```python
from build123d import *

# Parameters (mm, degrees)
EXTRUDE_11_REACH             = 60.31
EXTRUDE_11_DIRECTION_2_REACH = 60.31
CUT_EXTRUDE_1_DEPTH          = 7.5
CUT_EXTRUDE_1_DEPTH_BACK     = 7.5
CUT_EXTRUDE_2_DEPTH          = 5
CUT_EXTRUDE_START            = 28.688718626
CUT_EXTRUDE_3_DEPTH          = 1.311276176


# Read off the part's stored shape, not the designer's step: 切除-拉伸3
with BuildPart() as part:
    # 草图1 → 旋转1 (revolve)
    with BuildSketch(Plane.XY, mode=Mode.PRIVATE) as revolve_1_sk:
        Polygon((26.5, 38.4), (26.5, 36), (29, 36), (29, 0), (30, 0), (30, 40), (29, 40), (29, 38.4), align=None)
    revolve_1 = revolve(revolve_1_sk.sketch.rotate(Axis((0, 66, 0), (0, -1, 0)), 90), axis=Axis((0, 66, 0), (0, -1, 0)))

    # 镜向1: 旋转1 across plane
    add(revolve_1.mirror(Plane.ZX))

    # 凸台-拉伸11: up to this face of the body (flat: up to its plane)
    extrude_11_end = Plane(part.part.faces().sort_by_distance((0, 36, -27.320243866))[0])
    # 草图11 → 凸台-拉伸11 (add, up to the picked face)
    with BuildSketch(Plane(origin=(0, 0, 0), x_dir=(1, 0, 0), z_dir=(0, 1, 0)), mode=Mode.PRIVATE) as extrude_11_sk1:
        with BuildLine():
            Line((-13.076696831, -27), (13.076696831, -27))
            ThreePointArc((13.076696831, -27), (0, -30), (-13.076696831, -27))
        make_face()
    extrude_11_tool1 = split(extrude(extrude_11_sk1.sketch, amount=EXTRUDE_11_REACH, mode=Mode.PRIVATE), bisect_by=extrude_11_end, keep=Keep.BOTH, mode=Mode.PRIVATE)
    add(extrude_11_tool1.solids().sort_by(Axis((0, 0, 28.205296), (0, 1, 0)))[0])

    # 凸台-拉伸11 direction 2: up to this face of the body (flat: up to its plane)
    extrude_11_direction_2_end = Plane(part.part.faces().sort_by_distance((0, -36, -27.320243866))[0])
    # 草图11 → 凸台-拉伸11 direction 2 (add, up to the picked face)
    with BuildSketch(Plane(origin=(0, 0, 0), x_dir=(1, 0, 0), z_dir=(0, 1, 0)), mode=Mode.PRIVATE) as extrude_11_direction_2_sk1:
        with BuildLine():
            Line((-13.076696831, -27), (13.076696831, -27))
            ThreePointArc((13.076696831, -27), (0, -30), (-13.076696831, -27))
        make_face()
    extrude_11_direction_2_tool1 = split(extrude(extrude_11_direction_2_sk1.sketch, amount=-EXTRUDE_11_DIRECTION_2_REACH, mode=Mode.PRIVATE), bisect_by=extrude_11_direction_2_end, keep=Keep.BOTH, mode=Mode.PRIVATE)
    add(extrude_11_direction_2_tool1.solids().sort_by(Axis((0, 0, 28.205296), (0, -1, 0)))[0])

    # 草图12 → 切除-拉伸1 (cut, two sides: drawn at the far end of the back side and taken through both)
    with BuildSketch(Plane(origin=(0, 0, 0), x_dir=(1, 0, 0), z_dir=(0, 1, 0)).offset(-CUT_EXTRUDE_1_DEPTH_BACK)):
        with BuildLine():
            Line((0, 0), (22.520337054, 22.934948885))
            ThreePointArc((22.520337054, 22.934948885), (31.296937417, -7.32660697), (10, -30.547953473))
            Line((10, -30.547953473), (0, 0))
        make_face()
    extrude(amount=CUT_EXTRUDE_1_DEPTH + CUT_EXTRUDE_1_DEPTH_BACK, mode=Mode.SUBTRACT)

    # Sketch 3D_2 → 切除-拉伸2 (cut)
    with BuildSketch(Plane(origin=(35, 15, -4.993961669), x_dir=(-0.989973390659655, 0, 0.1412539761770484), z_dir=(0, 1, 0))):
        with BuildLine():
            Line((0, 0), (35.354485616, 0))
            Line((35.354485616, 0), (0.330334968, 4.976372773))
            ThreePointArc((0.330334968, 4.976372773), (0.075684949, 2.494126297), (0, 0))
        make_face()
    cut_extrude_2 = extrude(amount=CUT_EXTRUDE_2_DEPTH, mode=Mode.SUBTRACT)

    # 镜向2: 切除-拉伸2 across plane
    add(cut_extrude_2.mirror(Plane.ZX), mode=Mode.SUBTRACT)

    # 切除-拉伸3 outline → 切除-拉伸3 (cut)
    with BuildSketch(Plane.YZ.offset(CUT_EXTRUDE_START)):
        with BuildLine():
            Line((15, -4.237619285), (15, -0.017659399))
            add(Edge.make_bspline(
                [(15, -0.017659399), (12.884666816, -0.017659399), (12.884666816, -2.127639342), (12.884666816, -4.237619285), (15, -4.237619285)],
                knots=[3.141592654, 3.141592654, 3.141592654, 4.71238898, 4.71238898, 6.283185307, 6.283185307, 6.283185307], degree=2, weights=[1, 0.707106781, 1, 0.707106781, 1]))
        make_face()
    cut_extrude_3 = extrude(amount=CUT_EXTRUDE_3_DEPTH, mode=Mode.SUBTRACT)

    # 镜向3: 切除-拉伸3 across plane
    add(cut_extrude_3.mirror(Plane.ZX), mode=Mode.SUBTRACT)


solid = part.part
```
Geometry: final body of the model. Coordinates: model frame, mm. A direction names the side the tool comes from. Give positions to 0.01 mm unless a question says otherwise; leave off trailing zeros. Write each loop counter-clockwise with the first axis right and the second up, starting at its lowest first coordinate (ties: lowest second). Pieces come first, ordered by that corner, then holes.
1. Section query B-B, the plane z = 7.5. Return loops of the section in (x, y), then the cut area to 3 significant figures.
2. Draft query along Y for faces 1 (the cylindrical face through (-26.274, 37.183, -3.45)), 2 (the flat face through (23.5, 38.4, 12.8)), 3 (the flat face through (6, 36, -26)). Return one class per face: released by +Y, released by -Y, zero draft, split by the parting line, or undercut.
3. Line query: probe 1 along X at (y, z) = (37, 0); probe 2 along Y at (x, z) = (14, 24.5); probe 3 along X at (y, z) = (-39, 0). Output: solid intervals per line, ascending.
4. Reachability of faces 4 (the cylindrical face through (-26.274, -37.183, -3.45)), 5 (the cylindrical face through (25.73, 39.19, 13.38)), 6 (the flat face through (0, 1, 27)), 7 (the flat face through (23.5, -38.4, 12.8)) from +Z, -Z, +X, -X, +Y, -Y: full face, straight path, thin tool, end or side. Return the list, or none.
5. Section query D-D, the plane x = -21.5. Return loops of the section in (y, z), then the cut area to 3 significant figures.
6. Section query C-C, the plane y = 6. Return loops of the section in (x, z), then the cut area to 3 significant figures.
7. Pin query (flat end, axial travel): P1, Ø12, axis at x = 14, y = -4.5, coming from the -Z side; P2, Ø4, axis at x = 21, y = -1, coming from the -Z side; P3, Ø1, axis at x = -13.5, y = -31, coming from the +Z side; P4, Ø17, axis at x = -2, y = -16.5, coming from the -Z side. Return the tip coordinate at first contact, or that it passes through.
8. Section query A-A, the plane x = 0. Return loops of the section in (y, z), then the cut area to 3 significant figures.
Computed:
1. outline: (-29.05, -40) - (-28.01, -40) - (-28.01, -38.4) - (-25.42, -38.4) - (-25.42, -36) - (-28.01, -36) - (-28.01, 36) - (-25.42, 36) - (-25.42, 38.4) - (-28.01, 38.4) - (-28.01, 40) - (-29.05, 40) - close; (25.42, -38.4) - (28.01, -38.4) - (28.01, -40) - (29.05, -40) - (29.05, -7.5) - (28.01, -7.5) - (28.01, -36) - (25.42, -36) - close; (25.42, 36) - (28.01, 36) - (28.01, 7.5) - (29.05, 7.5) - (29.05, 40) - (28.01, 40) - (28.01, 38.4) - (25.42, 38.4) - close
1. area: 175 mm2
2. face 1: zero draft
2. face 2: released by +Y
2. face 3: undercut
3. probe 1: x = -30 to -26.5, 26.5 to 30
3. probe 2: y = -38.4 to -36, 36 to 38.4
3. probe 3: x = -30 to -29, 29 to 30
4. face 4: +Y, -Y
4. face 5: +Y
4. face 6: none
4. face 7: -Y
5. outline: (-40, -20.92) - (40, -20.92) - (40, -19.46) - (38.4, -19.46) - (38.4, -15.49) - (36, -15.49) - (36, -19.46) - (-36, -19.46) - (-36, -15.49) - (-38.4, -15.49) - (-38.4, -19.46) - (-40, -19.46) - close; (-40, 19.46) - (-38.4, 19.46) - (-38.4, 15.49) - (-36, 15.49) - (-36, 19.46) - (36, 19.46) - (36, 15.49) - (38.4, 15.49) - (38.4, 19.46) - (40, 19.46) - (40, 20.92) - (-40, 20.92) - close
5. area: 272 mm2
6. outline: (-10.58, 27) - (8.84, 27) - (9.33, 28.51) arc R30 ccw (long way) to (21.02, -21.41) - (20.32, -20.69) arc R29 cw (long way) to start
6. area: 153 mm2
7. P1: stops at z = -28.91
7. P2: stops at z = -23.22
7. P3: stops at z = 27.04
7. P4: stops at z = -30
8. outline: (-40, -30) - (40, -30) - (40, -29) - (38.4, -29) - (38.4, -26.5) - (36, -26.5) - (36, -29) - (-36, -29) - (-36, -26.5) - (-38.4, -26.5) - (-38.4, -29) - (-40, -29) - close; (-40, 29) - (-38.4, 29) - (-38.4, 26.5) - (-36, 26.5) - (-36, 27) - (36, 27) - (36, 26.5) - (38.4, 26.5) - (38.4, 29) - (40, 29) - (40, 30) - (-40, 30) - close
8. area: 328 mm2
